Check sheet for the drawn part. Datum: minimum x, y, z corner. Units: mm. A direction names the side the tool comes from. Round coordinates to 2 decimals unless told otherwise and drop trailing zeros. Write each loop counter-clockwise with the first axis right and the second up, starting at its lowest first coordinate (ties: lowest second). Pieces come first, ordered by that corner, then holes. Notation, with made-up numbers: M 79.25,23.25 L 96.25,23.25 A27 cw 96.25,54.25 Z; hole C 26,3.5 d8. An arc over 180 degrees is marked long. Use a Markdown table: item, result.
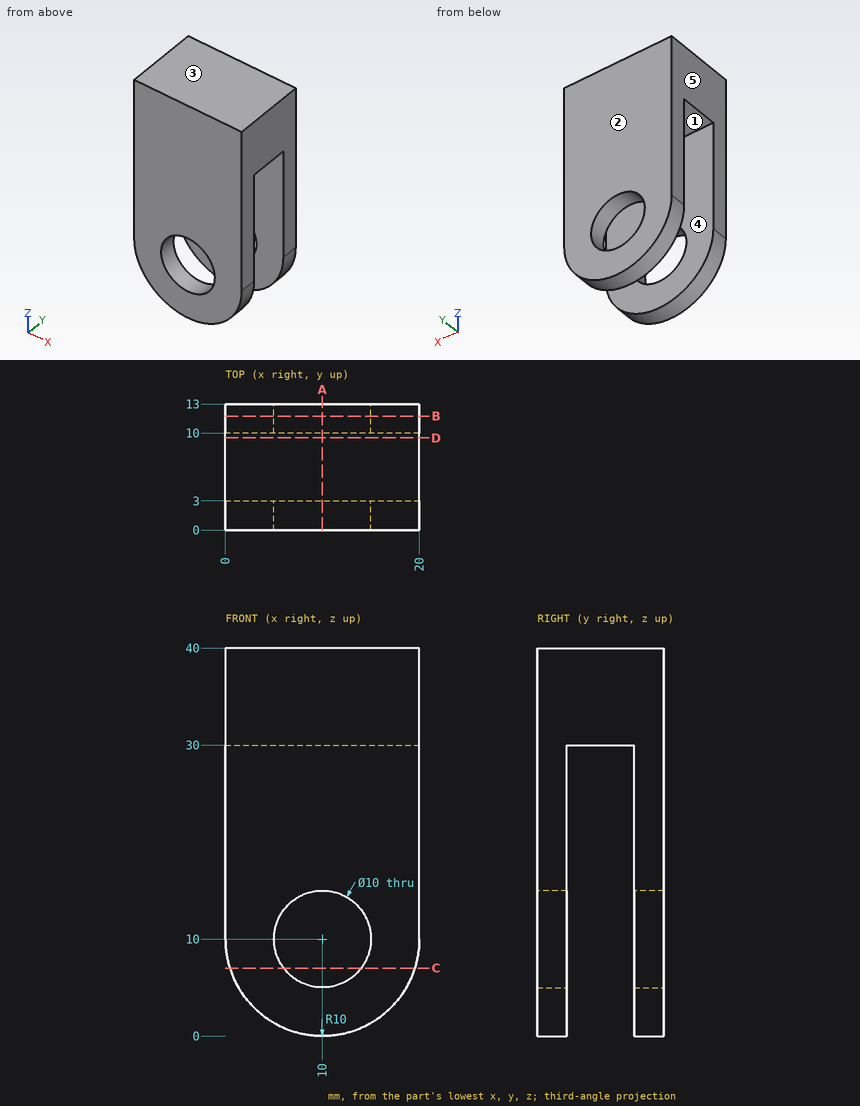
Item 1: Go/stop test with flat-tipped pins: pin 1 (6 mm diameter, centred on x = 9, y = 9, fed in from -Z); pin 2 (9 mm diameter, centred on x = 10, z = 10, fed in from +Y); pin 3 (3.5 mm diameter, centred on x = 9.5, y = 7, fed in from -Z); pin 4 (1.5 mm diameter, centred on x = 14, y = 9.5, fed in from -Z). Record where each tip stops, or that it passes through.
Outcome:
| item | result |
|---|---|
| pin 1 | stops at z = 0 |
| pin 2 | passes through |
| pin 3 | stops at z = 30 |
| pin 4 | stops at z = 0.61 |
Item 2: Mould release check, pull along Y, two halves, no side actions. Record for the marked faces 1, 2 and 3: +Y half, -Y half, draft (parallel to the pull), parting line (faces both ways), or undercut.
Outcome:
| item | result |
|---|---|
| face 1 | undercut |
| face 2 | +Y half |
| face 3 | draft |
Item 3: Material ranges on line 1 along Y through (x, z) = (6.25, 26.5); line 2 along X through (y, z) = (1.55, 10); line 3 along Z through (x, y) = (6.25, 7), recorded low to high. Write a range as from..to.
Outcome:
| item | result |
|---|---|
| line 1 | y = 0..3, 10..13 |
| line 2 | x = 0..5, 15..20 |
| line 3 | z = 30..40 |
Item 4: Cross-section at C-C, the plane z = 7. Record the cut outline in (x, y), and give its area (3 significant figures).
Outcome:
| item | result |
|---|---|
| outline | M 0.46,0 L 6,0 L 6,3 L 0.46,3 Z; M 0.46,10 L 6,10 L 6,13 L 0.46,13 Z; M 14,0 L 19.54,0 L 19.54,3 L 14,3 Z; M 14,10 L 19.54,10 L 19.54,13 L 14,13 Z |
| area | 66.5 mm2 |
Item 5: Cross-section at B-B, the plane y = 11.75. Record the cut outline in (x, z).
Outcome:
| item | result |
|---|---|
| outline | M 0,10 A10 ccw 20,10 L 20,40 L 0,40 Z; hole C 10,10 d10 |
Item 6: Access from +Z, -Z, +X, -X, +Y, -Y to the whole of each face (thin tool, end or side, straight path). Record for the marked faces 4 and 5.
Outcome:
| item | result |
|---|---|
| face 4 | -Z, +X, -X |
| face 5 | +Z, -Z, -X, +Y, -Y |
Item 7: Cross-section at A-A, the plane x = 10. Record the cut outline in (y, z).
Outcome:
| item | result |
|---|---|
| outline | M 0,0 L 3,0 L 3,5 L 0,5 Z; M 0,15 L 3,15 L 3,30 L 10,30 L 10,15 L 13,15 L 13,40 L 0,40 Z; M 10,0 L 13,0 L 13,5 L 10,5 Z |
Item 8: Cross-section at D-D, the plane y = 9.5. Record the cut outline in (x, z), and give its area (3 significant figures).
Outcome:
| item | result |
|---|---|
| outline | M 0,30 L 20,30 L 20,40 L 0,40 Z |
| area | 200 mm2 |
